Could you check a few things on this model? Use its own coordinates, in mm. A direction names the side the tool comes from. Give positions to 0.01 mm unless a question says otherwise; leave off trailing zeros. Write each loop counter-clockwise with the first axis right and the second up, starting at its lowest first coordinate (ties: lowest second). Pieces come first, ordered by that corner, then holes. Notation, with made-up numbers: (34.5, 34.5) - (62.5, 34.5) arc R19 cw to (62.5, 56.5) - close; hole circle Ø2 at (10, -7). An arc over 180 degrees is marked (long way). Answer as a JSON object with one key per item and string values. Group by question number.
```python
from build123d import *

# Parameters (mm, degrees)
PAD_DEPTH       = 15
SKETCH001_R     = 5
POCKET_DEPTH    = 21
SKETCH002_R     = 10
POCKET001_DEPTH = 40
FILLET_R        = 5
CHAMFER_SIZE    = 2
CHAMFER001_SIZE = 0.5
CHAMFER002_SIZE = 1
CHAMFER003_SIZE = 0.5
FILLET001_R     = 2


with BuildPart() as part:
    # Sketch → Pad (new body, symmetric)
    with BuildSketch(Plane.XZ):
        with BuildLine():
            Line((90, 0), (90, -14.746902))
            ThreePointArc((84.792982, -20.694269), (88.514305, -18.699249), (90, -14.746902))
            Line((84.792982, -20.694269), (20.207018, -29.305731))
            ThreePointArc((20.207018, -29.305731), (16.485695, -31.300751), (15, -35.253098))
            Line((15, -35.253098), (15, -60))
            Line((15, -60), (-15, -60))
            Line((-15, -60), (-15, -35.253098))
            ThreePointArc((-15, -35.253098), (-16.485695, -31.300751), (-20.207018, -29.305731))
            Line((-20.207018, -29.305731), (-84.792982, -20.694269))
            ThreePointArc((-90, -14.746902), (-88.514305, -18.699249), (-84.792982, -20.694269))
            Line((-90, -14.746902), (-90, 0))
            Line((-90, 0), (0, 0))
            Line((0, 0), (90, 0))
        make_face()
    extrude(amount=PAD_DEPTH, both=True)

    # Sketch001 (on Face14 of Pad) → Pocket (cut)
    with BuildSketch(Plane(origin=(0, 0, 0), x_dir=(-1, 0, 0), z_dir=(0, 0, 1))):
        with Locations((-45, 0)):
            Circle(SKETCH001_R)
        with Locations((45, 0)):
            Circle(SKETCH001_R)
    extrude(amount=-POCKET_DEPTH, mode=Mode.SUBTRACT)

    # Sketch002 (on Face14 of Pocket) → Pocket001 (cut)
    with BuildSketch(Plane(origin=(0, 0, -60), x_dir=(1, 0, 0), z_dir=(0, 0, -1))):
        Circle(SKETCH002_R)
    extrude(amount=-POCKET001_DEPTH, mode=Mode.SUBTRACT)

    # Fillet
    fillet_edges = [part.edges().sort_by_distance(p)[0] for p in [
        (90, -15, -7.373451),
        (-90, -15, -7.373451),
        (-90, 15, -7.373451),
        (90, 15, -7.373451),
    ]]
    fillet(fillet_edges, radius=FILLET_R)

    # Chamfer
    chamfer_edges = [part.edges().sort_by_distance(p)[0] for p in [
        (-10, 0, -60),
    ]]
    chamfer(chamfer_edges, length=CHAMFER_SIZE)

    # Chamfer001
    chamfer001_edges = [part.edges().sort_by_distance(p)[0] for p in [
        (-10, 0, -20),
    ]]
    chamfer(chamfer001_edges, length=CHAMFER001_SIZE)

    # Chamfer002
    chamfer002_edges = [part.edges().sort_by_distance(p)[0] for p in [
        (-40, 0, 0),
        (50, 0, 0),
    ]]
    chamfer(chamfer002_edges, length=CHAMFER002_SIZE)

    # Chamfer003
    chamfer003_edges = [part.edges().sort_by_distance(p)[0] for p in [
        (50, 0, -21),
        (-40, 0, -21),
    ]]
    chamfer(chamfer003_edges, length=CHAMFER003_SIZE)

    # Fillet001
    fillet001_edges = [part.edges().sort_by_distance(p)[0] for p in [
        (0, -15, -60),
    ]]
    fillet(fillet001_edges, radius=FILLET001_R)


solid = part.part
```
(1) I need wall thicknesses on L1, parallel to X at y = 0, z = -8.75; L2, parallel to Y at x = 45, z = -7.25; L3, parallel to X at y = -3, z = -41. Which ranges of each line are inside material? Lowest first, please.
(2) For faces 1 (the cylindrical face through (14, 13, -47)), 2 (the flat face through (-15, 0, -47)), 3 (the flat face through (45, 0, -21)), 4 (the flat face through (0, 0, -20)), which set-ups out of +Z, -Z, +X, -X, +Y, -Y let a thin tool reach every point of the face, with its end or its side?
(3) Will these pins go through, and if not, where does the flat tip stop? P1, Ø2.5, axis at x = 46, y = -2, coming from the +Z side; P2, Ø9, axis at x = -45, y = 0, coming from the -Z side; P3, Ø16, axis at y = 0.5, z = -45.5, coming from the +X side.
(4) I want a section at B-B, the plane x = 0. Please give me the cut outline in (y, z), and give its area (3 significant figures).
(5) I want a section at A-A, the plane z = -42. Please give me the cut outline in (x, y).
(6) If we mould it in two halves opening along Y, with no side actions, what happens to faces 5 (the cylindrical face through (-40, 0, -11)), 6 (the cylindrical face through (-13, -14, -46)), 7 (the flat face through (15, 0, -46))? For each: +Y half, -Y half, draft (parallel to the pull), parting line (faces both ways), or undercut.
Entries:
{
 "1": {"L1": "-90 to -50, -40 to 40, 50 to 90", "L2": "-15 to -5, 5 to 15", "L3": "-15 to -9.54, 9.54 to 15"},
 "2": {"face 1": "-Z, +X, +Y", "face 2": "-Z, -X, +Y, -Y", "face 3": "+Z", "face 4": "-Z"},
 "3": {"P1": "z = -21", "P2": "z = -26.6", "P3": "x = 15"},
 "4": {"outline": "(-15, -58) arc R2 ccw to (-13, -60) - (-12, -60) - (-10, -58) - (-10, -20.5) - (-9.5, -20) - (9.5, -20) - (10, -20.5) - (10, -58) - (12, -60) - (13, -60) arc R2 ccw to (15, -58) - (15, 0) - (-15, 0) - close", "area": "995 mm^2"},
 "5": {"outline": "(-15, -10) arc R5 ccw to (-10, -15) - (10, -15) arc R5 ccw to (15, -10) - (15, 10) arc R5 ccw to (10, 15) - (-10, 15) arc R5 ccw to (-15, 10) - close; hole circle Ø20 at (0, 0)"},
 "6": {"face 5": "undercut", "face 6": "-Y half", "face 7": "draft"}
}
